```python
from build123d import *

# Parameters (mm, degrees)
F3_R = 5


with BuildPart() as f2:
    # F2: sweep along a path in F1
    with BuildLine(Plane.YZ) as f2_path:
        Line((0, 0), (0, 30))
        Line((0, 30), (-38.5672565812, 75.9626665871))
        Line((-38.5672565812, 75.9626665871), (-68.5672565812, 81.2524760084))
    # F0 (on Top) → F2 (sweep)
    with BuildSketch(Plane.XY):
        with BuildLine():
            Line((-10, 15), (-20, 15))
            Line((-20, 15), (-20, -15))
            Line((-20, -15), (20, -15))
            Line((20, -15), (20, 15))
            Line((20, 15), (10, 15))
            add(Edge.make_bspline(
                [(10, 15), (11.0915185913, 13.5177812127), (13.4276997431, 10.3453830316), (15.1647077967, 2.8381597184), (10.8372280842, -6.6356174494), (3.701873231, -8.2492537512), (0, -9.0864198282)],
                knots=[0, 0, 0, 0, 0.2084843189, 0.4462197347, 0.7126948299, 1, 1, 1, 1], degree=3))
            add(Edge.make_bspline(
                [(-10, 15), (-11.0915185913, 13.5177812127), (-13.4276997431, 10.3453830316), (-15.1647077967, 2.8381597184), (-10.8372280842, -6.6356174494), (-3.701873231, -8.2492537512), (0, -9.0864198282)],
                knots=[0, 0, 0, 0, 0.2084843189, 0.4462197347, 0.7126948299, 1, 1, 1, 1], degree=3))
        make_face()
    sweep(path=f2_path.line, transition=Transition.RIGHT)

    # F3
    f3_edges = [f2.edges().sort_by_distance(p)[0] for p in [
        (-20, -7.792962, 62.623147),
        (-20, 15, 17.729777),
        (-20, -15, 12.270223),
        (-20, -30.774295, 43.339519),
        (-20, -58.860285, 64.309476),
        (-20, -68.567257, 81.252476),
        (-20, -48.274229, 92.905667),
        (20, -7.792962, 62.623147),
        (20, 15, 17.729777),
        (20, -48.274229, 92.905667),
        (20, 0, 0),
        (20, -15, 12.270223),
        (20, -30.774295, 43.339519),
        (20, -58.860285, 64.309476),
        (20, -68.567257, 81.252476),
        (15, -65.962534, 96.024592),
        (-15, -65.962534, 96.024592),
        (0, -71.171979, 66.48036),
        (0, -15, 0),
        (-15, 15, 0),
        (15, 15, 0),
    ]]
    fillet(f3_edges, radius=F3_R)


solid = f2.part
```
Source: CAD feature listing. Evaluate the final solid. Frame: model axes, mm. A direction names the side the tool comes from. Give positions to 0.01 mm unless a question says otherwise; leave off trailing zeros. Loops run counter-clockwise (first coordinate to the right, second up) from the corner with the lowest first, then second, coordinate; pieces in that order, holes last. Notation, with made-up numbers: (24.5, 80) -> (45.5, 80) arc R16 cw to (45.5, 92) -> close; hole circle Ø4 at (47.5, 41.5). An arc over 180 degrees is marked (long way). Use a Markdown table: item, result. Add a question column.
(1) Access query for faces 1 (the face through (-19, -13, 13)), 2 (the face through (18.57, -9.26, 62.04)). Directions: +Z, -Z, +X, -X, +Y, -Y. A direction counts if a zero-diameter tool reaches every point of the face in a straight line with its end or side. Return the directions, or none.
(2) First-contact query: pin 1 Ø5 at (y, z) = (-33, 47.5) entering from -X; pin 2 Ø6 at (x, y) = (-16, -47) entering from -Z; pin 3 Ø6 at (x, z) = (2.5, 15) entering from -Y. Flat tips, straight axial feed; report the tip coordinate or a pass-through.
(3) Ray query, line 1 (X direction, y = -6, z = 14); line 2 (Z direction, x = 11.5, y = -11); line 3 (Y direction, x = 11, z = 31). Return the intervals inside material, ascending.
(4) Section query A-A (x = 17). Output: boundary loops of the cut face in (y, z).
(5) Section query B-B (x = -17). Output: boundary loops of the cut face in (y, z), then the cut area to 3 significant figures.
Checked values:
| question | item | result |
|---|---|---|
| 1 | face 1 | -Z, -X, -Y |
| 1 | face 2 | +Z, +X, +Y |
| 2 | pin 1 | x = -19.76 |
| 2 | pin 2 | z = 59.19 |
| 2 | pin 3 | y = -15 |
| 3 | line 1 | -20 to -8.95, 8.95 to 20 |
| 3 | line 2 | 0.1 to 37.4, 63.17 to 66.45 |
| 3 | line 3 | -20.42 to -6.4, 13.62 to 15 |
| 4 | outline | (-69.89, 71.33) arc R4.58 ccw to (-66.18, 66.02) -> (-46.33, 62.52) -> (-14.58, 24.69) -> (-14.58, 5) arc R4.58 ccw to (-10, 0.42) -> (10, 0.42) arc R4.58 ccw to (14.58, 5) -> (14.58, 35.31) -> (-30.81, 89.4) -> (-61.11, 94.75) arc R4.58 ccw to (-66.42, 91.03) -> close |
| 5 | outline | (-69.89, 71.33) arc R4.58 ccw to (-66.18, 66.02) -> (-46.33, 62.52) -> (-14.58, 24.69) -> (-14.58, 3) arc R5 ccw to (-10, 0) -> (10, 0) arc R5 ccw to (14.58, 3) -> (14.58, 35.31) -> (-30.81, 89.4) -> (-61.11, 94.75) arc R4.58 ccw to (-66.42, 91.03) -> close |
| 5 | area | 3,480 mm^2 |
